from build123d import *

# Parameters (mm, degrees)
SKETCH1_R           = 2.1
BOSS_EXTRUDE1_DEPTH = 7


with BuildPart() as part:
    # Sketch1 → Boss-Extrude1 (new body)
    with BuildSketch(Plane.XY):
        with BuildLine():
            Line((0.5, 3.968626967), (0, 3.468626967))
            Line((0, 3.468626967), (-0.5, 3.968626967))
            ThreePointArc((-0.5, 3.968626967), (-1.236067977, 3.804226065), (-1.928191906, 3.504579286))
            Line((-1.928191906, 3.504579286), (-2.038807777, 2.806178163))
            Line((-2.038807777, 2.806178163), (-2.7372089, 2.916794034))
            ThreePointArc((-2.7372089, 2.916794034), (-3.236067977, 2.351141009), (-3.61988004, 1.701901435))
            Line((-3.61988004, 1.701901435), (-3.298860279, 1.07186468))
            Line((-3.298860279, 1.07186468), (-3.928897035, 0.750844919))
            ThreePointArc((-3.928897035, 0.750844919), (-4, 0), (-3.928897035, -0.750844919))
            Line((-3.928897035, -0.750844919), (-3.298860279, -1.07186468))
            Line((-3.298860279, -1.07186468), (-3.61988004, -1.701901435))
            ThreePointArc((-3.61988004, -1.701901435), (-3.236067977, -2.351141009), (-2.7372089, -2.916794034))
            Line((-2.7372089, -2.916794034), (-2.038807777, -2.806178163))
            Line((-2.038807777, -2.806178163), (-1.928191906, -3.504579286))
            ThreePointArc((-1.928191906, -3.504579286), (-1.236067977, -3.804226065), (-0.5, -3.968626967))
            Line((-0.5, -3.968626967), (0, -3.468626967))
            Line((0, -3.468626967), (0.5, -3.968626967))
            ThreePointArc((0.5, -3.968626967), (1.236067977, -3.804226065), (1.928191906, -3.504579286))
            Line((1.928191906, -3.504579286), (2.038807777, -2.806178163))
            Line((2.038807777, -2.806178163), (2.7372089, -2.916794034))
            ThreePointArc((2.7372089, -2.916794034), (3.236067977, -2.351141009), (3.61988004, -1.701901435))
            Line((3.61988004, -1.701901435), (3.298860279, -1.07186468))
            Line((3.298860279, -1.07186468), (3.928897035, -0.750844919))
            ThreePointArc((3.928897035, -0.750844919), (4, 0), (3.928897035, 0.750844919))
            Line((3.928897035, 0.750844919), (3.298860279, 1.07186468))
            Line((3.298860279, 1.07186468), (3.61988004, 1.701901435))
            ThreePointArc((3.61988004, 1.701901435), (3.236067977, 2.351141009), (2.7372089, 2.916794034))
            Line((2.7372089, 2.916794034), (2.038807777, 2.806178163))
            Line((2.038807777, 2.806178163), (1.928191906, 3.504579286))
            ThreePointArc((1.928191906, 3.504579286), (1.236067977, 3.804226065), (0.5, 3.968626967))
        make_face()
        Circle(SKETCH1_R, mode=Mode.SUBTRACT)
    extrude(amount=BOSS_EXTRUDE1_DEPTH)


solid = part.part
Input: part model. Units: mm. Frame: model coordinates. Give positions to 0.01 mm unless a question says otherwise; leave off trailing zeros. Write each loop counter-clockwise with the first axis right and the second up, starting at its lowest first coordinate (ties: lowest second). Pieces come first, ordered by that corner, then holes.
Q1. Section D-D, the plane y = -2.5. Output: boundary loops of the cut face in (x, z), plus the area to 3 significant figures.
Q2. Material intervals for probe 1 along Y at (x, z) = (1.75, 5); probe 2 along X at (y, z) = (3.25, 5.5), sorted ascending.
Q3. Pull-direction query (X, two-part tool) for faces 1 (the face through (2.003, 0.631, 3.451)), 2 (the face through (3.2, -2.4, 3.5)), 3 (the face through (2, -2, 0)), 4 (the face through (-1.25, -3.8, 3.45)); classes: pulls with the +X half, pulls with the -X half, needs draft (parallel to the pull), parting line crosses it, or undercut.
Q4. Section C-C, the plane x = 1.25. Output: boundary loops of the cut face in (y, z), plus the area to 3 significant figures.
Q5. First-contact query: P1, Ø4, axis at x = -3, z = 3.5, coming from the -Y side; P2, Ø2, axis at y = 2.5, z = 6, coming from the -X side. Flat tips, straight axial feed; report the tip coordinate or a pass-through.
Q6. Section A-A, the plane y = 0. Output: boundary loops of the cut face in (x, z), plus the area to 3 significant figures.
Filled in:
1. outline: (-3.12, 0) - (3.12, 0) - (3.12, 7) - (-3.12, 7) - close
1. area: 43.7 mm2
2. probe 1: y = -3.6 to -1.16, 1.16 to 3.6
2. probe 2: x = -1.97 to 1.97
3. face 1: undercut
3. face 2: pulls with the +X half
3. face 3: needs draft
3. face 4: pulls with the -X half
4. outline: (-3.8, 0) - (-1.69, 0) - (-1.69, 7) - (-3.8, 7) - close; (1.69, 0) - (3.8, 0) - (3.8, 7) - (1.69, 7) - close
4. area: 29.6 mm2
5. P1: stops at y = -3.87
5. P2: stops at x = -3.62
6. outline: (-4, 0) - (-2.1, 0) - (-2.1, 7) - (-4, 7) - close; (2.1, 0) - (4, 0) - (4, 7) - (2.1, 7) - close
6. area: 26.6 mm2
